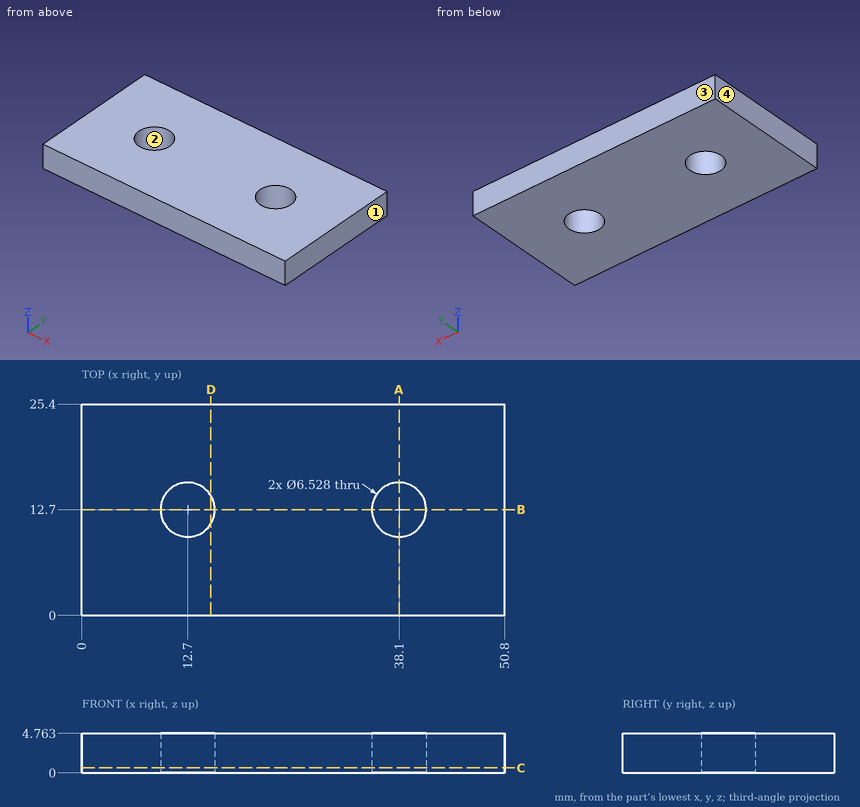
Design review of the part shown in the three views and the two pictorial views. Dimensions are in mm from the part's minimum x, y and z. Round coordinates to 2 decimals unless told otherwise and drop trailing zeros. Loops run counter-clockwise (first coordinate to the right, second up) from the corner with the lowest first, then second, coordinate; pieces in that order, holes last. Notation, with made-up numbers: (48, 60) -> (107, 60) arc R12 ccw to (107, 72) -> close; hole circle Ø7 at (73.5, 59.5). An arc over 180 degrees is marked (long way). Return JSON: item names as keys, results as strings.
(1) For line 1 (Y direction, x = 38.1, z = 3.25); line 2 (X direction, y = 10, z = 0.45) (1 decimal); line 3 (X direction, y = 14, z = 2.85) (1 decimal), list the stretches that pass through material, from the lowest coordinate up.
Solved:
{"line 1": "0 to 9.44, 15.96 to 25.4", "line 2": "0 to 10.9, 14.5 to 36.3, 39.9 to 50.8", "line 3": "0 to 9.7, 15.7 to 35.1, 41.1 to 50.8"}
(2) Add section B-B on y = 12.7. Write out the cut boundary in (x, z).
Solved:
{"outline": "(0, 0) -> (9.44, 0) -> (9.44, 4.76) -> (0, 4.76) -> close; (15.96, 0) -> (34.84, 0) -> (34.84, 4.76) -> (15.96, 4.76) -> close; (41.36, 0) -> (50.8, 0) -> (50.8, 4.76) -> (41.36, 4.76) -> close"}
(3) The part is to be moulded in two halves that separate along X. For the marked faces 1, 2, 3 and 4, say which applies: released by +X, released by -X, zero draft, split by the parting line, or undercut.
Solved:
{"face 1": "released by +X", "face 2": "undercut", "face 3": "zero draft", "face 4": "released by -X"}
(4) Add section D-D on x = 15.5. Write out the cut boundary in (y, z).
Solved:
{"outline": "(0, 0) -> (11.02, 0) -> (11.02, 4.76) -> (0, 4.76) -> close; (14.38, 0) -> (25.4, 0) -> (25.4, 4.76) -> (14.38, 4.76) -> close"}
(5) Add section C-C on z = 0.6. Write out the cut boundary in (x, y), plus the area to 3 significant figures.
Solved:
{"outline": "(0, 0) -> (50.8, 0) -> (50.8, 25.4) -> (0, 25.4) -> close; hole circle Ø6.53 at (12.7, 12.7); hole circle Ø6.53 at (38.1, 12.7)", "area": "1,220 mm2"}
(6) For pin 1 (7.5 mm diameter, centred on x = 38.1, y = 12.7, fed in from -Z), flat-tipped, find the tip position at first contact; note if it passes through.
Solved:
{"pin 1": "z = 0"}
(7) Add section A-A on x = 38.1. Write out the cut boundary in (y, z).
Solved:
{"outline": "(0, 0) -> (9.44, 0) -> (9.44, 4.76) -> (0, 4.76) -> close; (15.96, 0) -> (25.4, 0) -> (25.4, 4.76) -> (15.96, 4.76) -> close"}
